Part model, mm, in its own coordinate system. Round coordinates to 2 decimals unless told otherwise and drop trailing zeros. Loops run counter-clockwise (first coordinate to the right, second up) from the corner with the lowest first, then second, coordinate; pieces in that order, holes last. Notation, with made-up numbers: M -22.5,57.25 L 9.5,57.25 A19 cw 9.5,63.25 Z; hole C 8.5,-39.75 d8. An arc over 180 degrees is marked long. Put each result on its own line as item: value. Start each with the question number.
1) Slice it at B-B on x = -180. Give the cut face in (y, z), then the cut area to 3 significant figures.
2) Drop a flat-ended pin along its axis: pin 1 Ø24 at (x, y) = (-180, 0) entering from -Z. Give the stop position or say it passes through.
3) Probe line 1 along Y through (x, z) = (-180, 22.75); line 2 along X through (y, z) = (0.5, 7); line 3 along X through (y, z) = (-3, 4.75). List the from-to ranges inside material, lowest first.
4) Slice it at A-A on y = 0. Give the cut face in (x, z), then the cut area to 3 significant figures.
5) Pull direction Y, two halves, no side cores. Call faces 1 (the cylindrical face through (-194.985, -0.66, 14.79)), 2 (the flat face through (-4, 50, 15)), 3 (the flat face through (-4, 1, 0)), 4 (the flat face through (4, -50, 15)): +Y half, -Y half, draft (parallel to the pull), parting line (faces both ways), or undercut.
Autodesk Inventor part; units mm, degrees
ref_plane "YZ Plane" through (0, 0, 0) normal (1, 0, 0) x (0, 1, 0)
ref_plane "XZ Plane" through (0, 0, 0) normal (0, 1, 0) x (-1, 0, 0)
ref_plane "XY Plane" through (0, 0, 0) normal (0, 0, 1) x (1, 0, 0)
sketch "Эскиз1" plane through (0, 0, 0) normal (0, 0, 1) x (1, 0, 0)
  line L0 (300, -50) -> (-300, -50)
  line L1 (-300, -50) -> (-300, 50)
  line L2 (-300, 50) -> (300, 50)
  line L3 (300, 50) -> (300, -50)
  line L4 (300, -50) -> (-300, 50) construction
  line L5 (-300, -50) -> (300, 50) construction
  circle A0 centre (-180, 0) radius 15
  point P0 (0, 0)
  dimension "d0" = 100
  dimension "d1" = 600
  dimension "d4" = 30
  dimension "d5" = 120
extrude "Выдавливание1" add sketch "Эскиз1" along normal blind 30
properties material "Сталь, литейная"
Recorded:
1. outline: M -50,0 L -15,0 L -15,30 L -50,30 Z; M 15,0 L 50,0 L 50,30 L 15,30 Z
1. area: 2,100 mm2
2. pin 1: passes through
3. line 1: y = -50 to -15, 15 to 50
3. line 2: x = -300 to -194.99, -165.01 to 300
3. line 3: x = -300 to -194.7, -165.3 to 300
4. outline: M -300,0 L -195,0 L -195,30 L -300,30 Z; M -165,0 L 300,0 L 300,30 L -165,30 Z
4. area: 17,100 mm2
5. face 1: undercut
5. face 2: +Y half
5. face 3: draft
5. face 4: -Y half
